```python
from build123d import *

# Parameters (mm, degrees)
SKETCH2_R          = 3
CUT_EXTRUDE1_DEPTH = 24.184046239
CHAMFER1_SIZE      = 1.5


with BuildPart() as part:
    # Sketch1 → Revolve1 (revolve)
    with BuildSketch(Plane(origin=(0, 0, 0), x_dir=(1, 0, 0), z_dir=(0, 1, 0)), mode=Mode.PRIVATE) as revolve1_sk:
        Polygon((0, 7.5), (12.5, 7.5), (12.5, 5.5), (10, 5.5), (10, -5.5), (12.5, -5.5), (12.5, -7.5), (0, -7.5), align=None)
    revolve(revolve1_sk.sketch.rotate(Axis((0, 0, -16.700819672), (0, 0, 1)), 180), axis=Axis((0, 0, -16.700819672), (0, 0, 1)))

    # Sketch2 → Cut-Extrude1 (cut, through all)
    with BuildSketch(Plane(origin=(0, 0, -7.5), x_dir=(-1, 0, 0), z_dir=(0, 0, -1))):
        Circle(SKETCH2_R)
    extrude(amount=-CUT_EXTRUDE1_DEPTH, mode=Mode.SUBTRACT)

    # Chamfer1
    chamfer1_edges = [part.edges().sort_by_distance(p)[0] for p in [
        (12.5, 0, -5.5),
        (12.5, 0, 5.5),
    ]]
    chamfer(chamfer1_edges, length=CHAMFER1_SIZE)


solid = part.part
```
Model file for the job. Use its own axes, mm. A direction names the side the tool comes from. Give positions to 0.01 mm unless a question says otherwise; leave off trailing zeros. Loops run counter-clockwise (first coordinate to the right, second up) from the corner with the lowest first, then second, coordinate; pieces in that order, holes last. Notation, with made-up numbers: (16.25, 11.25) -> (49.25, 11.25) arc R34 cw to (49.25, 44.25) -> close; hole circle Ø8 at (-11.5, -1.75). An arc over 180 degrees is marked (long way). Write each question's results on one line, items separated by ' | '.
(1) Flat gauge pins, fed straight in: pin 1 Ø4 at (x, z) = (-0.5, -2) entering from +Y; pin 2 Ø5 at (x, z) = (-2.5, -5.5) entering from +Y; pin 3 Ø1.5 at (x, z) = (8, 5) entering from +Y. Where does each tip first touch, or does it go through?
Geometry results:
pin 1: stops at y = 10 | pin 2: stops at y = 12.49 | pin 3: stops at y = 8.14
(2) Tool access for faces 1 (the flat face through (-3, 3, 7.5)), 2 (the cylindrical face through (10, 0, 0)): list every direction of +Z, -Z, +X, -X, +Y, -Y with a clear straight run to the whole face (end or side of a thin tool).
Geometry results:
face 1: +Z, +X, -X, +Y, -Y | face 2: none
(3) Probe line 1 along Y through (x, z) = (0, 3.25); line 2 along Z through (x, y) = (-10, -1.25); line 3 along X through (y, z) = (-2, 6). List the from-to ranges inside material, lowest first.
Geometry results:
line 1: y = -10 to -3, 3 to 10 | line 2: z = -7.5 to -5.5, 5.5 to 7.5 | line 3: x = -11.32 to -2.24, 2.24 to 11.32
(4) Cut at C-C on z = 4.25. List the corners of the cut face in (x, y), and give its area (3 significant figures).
Geometry results:
outline: circle Ø20 at (0, 0); hole circle Ø6 at (0, 0) | area: 286 mm²
(5) Pull direction X, two halves, no side cores. Call faces 3 (the flat face through (-2, 10, -5.5)), 4 (the cylindrical face through (-11.923, -3.755, -7.246)), 5 (the cylindrical face through (3, 0, 0)): released by +X, released by -X, zero draft, split by the parting line, or undercut.
Geometry results:
face 3: zero draft | face 4: split by the parting line | face 5: undercut
(6) Cut at A-A on x = 0. List the corners of the cut face in (y, z), and give its area (4 significant figures).
Geometry results:
outline: (-12.5, -7.5) -> (-3, -7.5) -> (-3, 7.5) -> (-12.5, 7.5) -> (-12.5, 7) -> (-11, 5.5) -> (-10, 5.5) -> (-10, -5.5) -> (-11, -5.5) -> (-12.5, -7) -> close; (3, -7.5) -> (12.5, -7.5) -> (12.5, -7) -> (11, -5.5) -> (10, -5.5) -> (10, 5.5) -> (11, 5.5) -> (12.5, 7) -> (12.5, 7.5) -> (3, 7.5) -> close | area: 225.5 mm²
